```python
from build123d import *

# Parameters (mm, degrees)
F0_W     = 74
F0_H     = 66.5
F1_DEPTH = 1.6
F2_R     = 3
F3_R     = 2
F3_W     = 50
F3_H     = 17
F3_R_2   = 1.65
F4_DEPTH = 25


with BuildPart() as f1:
    # F0 (on Top) → F1 (new body)
    with BuildSketch(Plane.XY):
        with Locations((9.5, 9)):
            Rectangle(F0_W, F0_H)
    extrude(amount=F1_DEPTH)

    # F2
    f2_edges = [f1.edges().sort_by_distance(p)[0] for p in [
        (-27.5, 42.25, 0.8),
        (46.5, 42.25, 0.8),
    ]]
    fillet(f2_edges, radius=F2_R)

    # F3 (on face) → F4 (cut)
    with BuildSketch(Plane.XY.offset(1.6)):
        with Locations((-21, 19)):
            Circle(F3_R)
        with Locations((22, -19)):
            Circle(F3_R)
        with Locations((0, 5.25)):
            Rectangle(F3_W, F3_H)
        with Locations((-1.6, 37.127893)):
            Circle(F3_R_2)
        with Locations((11.1, 37.127893)):
            Circle(F3_R_2)
        with Locations((14.6, 37.127893)):
            Circle(F3_R_2)
        with Locations((27.3, 37.127893)):
            Circle(F3_R_2)
        with Locations((30.8, 37.127893)):
            Circle(F3_R_2)
        with Locations((43.5, 37.127893)):
            Circle(F3_R_2)
    extrude(amount=-F4_DEPTH, mode=Mode.SUBTRACT)


solid = f1.part
```
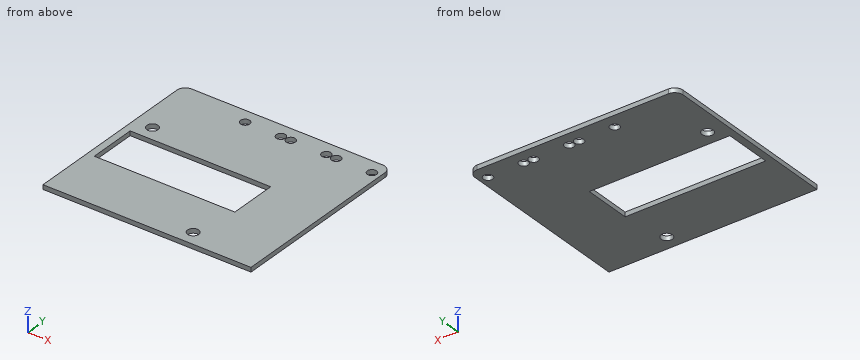
For this review, take the finished solid that the model builds, in its own axes (mm). Coordinates: 2 decimals unless noted, no trailing zeros. Loops run counter-clockwise (first coordinate to the right, second up) from the corner with the lowest first, then second, coordinate; pieces in that order, holes last.
1. For line 1 (Y direction, x = -21, z = 0.5); line 2 (Y direction, x = -16.5, z = 0.85); line 3 (X direction, y = 10.5, z = 0.6), list the stretches that pass through material, from the lowest coordinate up.
2. Add section B-B, the plane y = 19. Give the boundary of the cut face in (x, z), then the cut area to 3 significant figures.
3. Add section A-A, the plane x = -16. Give the boundary of the cut face in (y, z).
4. Add section C-C, the plane x = 14.6. Give the boundary of the cut face in (y, z).
5. Add section D-D, the plane z = 1.2. Count the separate pieces of the cut face and the enclosed holes in it, then the cut area to 3 significant figures.
Result:
1. line 1: y = -24.25 to -3.25, 13.75 to 17, 21 to 42.25
1. line 2: y = -24.25 to -3.25, 13.75 to 42.25
1. line 3: x = -27.5 to -25, 25 to 46.5
2. outline: (-27.5, 0) - (-23, 0) - (-23, 1.6) - (-27.5, 1.6) - close; (-19, 0) - (46.5, 0) - (46.5, 1.6) - (-19, 1.6) - close
2. area: 112 mm2
3. outline: (-24.25, 0) - (-3.25, 0) - (-3.25, 1.6) - (-24.25, 1.6) - close; (13.75, 0) - (42.25, 0) - (42.25, 1.6) - (13.75, 1.6) - close
4. outline: (-24.25, 0) - (-3.25, 0) - (-3.25, 1.6) - (-24.25, 1.6) - close; (13.75, 0) - (35.48, 0) - (35.48, 1.6) - (13.75, 1.6) - close; (38.78, 0) - (42.25, 0) - (42.25, 1.6) - (38.78, 1.6) - close
5. separate pieces: 1
5. enclosed holes: 9
5. area: 3,990 mm2
